Build history of the part. All positions in model axes, mm. A direction names the side the tool comes from. Give positions to 0.01 mm unless a question says otherwise; leave off trailing zeros. Loops run counter-clockwise (first coordinate to the right, second up) from the corner with the lowest first, then second, coordinate; pieces in that order, holes last.
1) Band-saw the part on C-C on x = 12. List the corners of the cut face in (y, z), then the cut area to 3 significant figures.
2) Band-saw the part on B-B on y = 108. List the corners of the cut face in (x, z).
3) Band-saw the part on A-A on z = 2. List the corners of the cut face in (x, y).
4) 3-axis set-ups, long thin cutter, end or side, ignore diameter. For faces 1 (the flat face through (24, 133, 4)), 2 (the cylindrical face through (12.1, 122.5, 9.5)), 3 (the flat face through (1, 73, 3)): which of +Z, -Z, +X, -X, +Y, -Y reach the whole face in a straight line?
5) Flat gauge pins, fed straight in: P1, Ø12, axis at x = 17.5, y = 70, coming from the -Z side; P2, Ø1.1, axis at y = 81.5, z = 9.5, coming from the +X side; P3, Ø10, axis at x = 13.5, y = 60.5, coming from the -Z side. Where does each tip first touch, or does it go through?
6) Band-saw the part on D-D on y = 26. List the corners of the cut face in (x, z).
7) Wall check: line 1 (X direction, y = 26.5, z = 7); line 2 (X direction, y = 106, z = 6.25); line 3 (Z direction, x = 20, y = 104). Give the ranges that are in metal, low to high.
```python
from build123d import *

# Parameters (mm, degrees)
F0_W            = 24
F0_H            = 148
F1_DEPTH        = 10
F2_R            = 2
F3_W            = 22
F3_H            = 9
F4_DEPTH        = 148
F5_R            = 2
F7_DEPTH        = 1
F8_R            = 2
F9_R            = 2
F11_D           = 5
F11_CSINK_D     = 8
F11_CSINK_ANGLE = 90
F13_W           = 58.5735701025
F13_H           = 8
F14_DEPTH       = 1.2689491924


with BuildPart() as f1:
    # F0 (on Top) → F1 (new body)
    with BuildSketch(Plane.XY):
        with Locations((12, 74)):
            Rectangle(F0_W, F0_H)
    extrude(amount=F1_DEPTH)

    # F2
    f2_edges = [f1.edges().sort_by_distance(p)[0] for p in [
        (0, 74, 10),
    ]]
    fillet(f2_edges, radius=F2_R)

    # F3 (on face) → F4 (cut, through all)
    with BuildSketch(Plane.XZ):
        with Locations((12, 4.5)):
            Rectangle(F3_W, F3_H)
    extrude(amount=-F4_DEPTH, mode=Mode.SUBTRACT)

    # F5
    f5_edges = [f1.edges().sort_by_distance(p)[0] for p in [
        (1, 74, 9),
    ]]
    fillet(f5_edges, radius=F5_R)

    # F6 (on face) → F7 (cut, through all)
    with BuildSketch(Plane.XY.offset(10)):
        with BuildLine():
            Line((16.5, 57), (16.5, 118))
            ThreePointArc((16.5, 118), (12, 122.5), (7.5, 118))
            Line((7.5, 118), (7.5, 57))
            ThreePointArc((7.5, 57), (12, 52.5), (16.5, 57))
        make_face()
    extrude(amount=-F7_DEPTH, mode=Mode.SUBTRACT)

    # F8
    f8_edges = [f1.edges().sort_by_distance(p)[0] for p in [
        (24, 74, 10),
    ]]
    fillet(f8_edges, radius=F8_R)

    # F9
    f9_edges = [f1.edges().sort_by_distance(p)[0] for p in [
        (23, 74, 9),
    ]]
    fillet(f9_edges, radius=F9_R)

    # F11 (through all)
    with Locations(Plane.XY.offset(10)):
        with Locations((12, 138), (12, 40), (12, 10)):
            CounterSinkHole(F11_D / 2, F11_CSINK_D / 2, counter_sink_angle=F11_CSINK_ANGLE)

    # F13 (on face) → F14 (cut, through all)
    with BuildSketch(Plane.YZ.offset(24)):
        with Locations((89.2871636897, 4)):
            Rectangle(F13_W, F13_H)
    extrude(amount=-F14_DEPTH, mode=Mode.SUBTRACT)


solid = f1.part
```
Findings below:
1. outline: (0, 9) - (7, 9) - (6, 10) - (0, 10) - close; (13, 9) - (37, 9) - (36, 10) - (14, 10) - close; (43, 9) - (52.5, 9) - (52.5, 10) - (44, 10) - close; (122.5, 9) - (135, 9) - (134, 10) - (122.5, 10) - close; (141, 9) - (148, 9) - (148, 10) - (142, 10) - close
1. area: 57.0 mm2
2. outline: (0, 0) - (1, 0) - (1, 7) arc R2 cw to (3, 9) - (7.5, 9) - (7.5, 10) - (2, 10) arc R2 ccw to (0, 8) - close; (16.5, 9) - (21, 9) arc R2 cw to (22.73, 8) - (24, 8) arc R2 ccw to (22, 10) - (16.5, 10) - close
3. outline: (0, 0) - (1, 0) - (1, 148) - (0, 148) - close; (23, 0) - (24, 0) - (24, 60) - (23, 60) - close; (23, 118.57) - (24, 118.57) - (24, 148) - (23, 148) - close
4. face 1: +Z, -Z, +X, +Y, -Y
4. face 2: +Z, -Z
4. face 3: -Z, +Y, -Y
5. P1: stops at z = 8
5. P2: stops at x = 23.76
5. P3: stops at z = 9
6. outline: (0, 0) - (1, 0) - (1, 7) arc R2 cw to (3, 9) - (21, 9) arc R2 cw to (23, 7) - (23, 0) - (24, 0) - (24, 8) arc R2 ccw to (22, 10) - (2, 10) arc R2 ccw to (0, 8) - close
7. line 1: x = 0 to 1, 23 to 24
7. line 2: x = 0 to 1
7. line 3: z = 9 to 10
